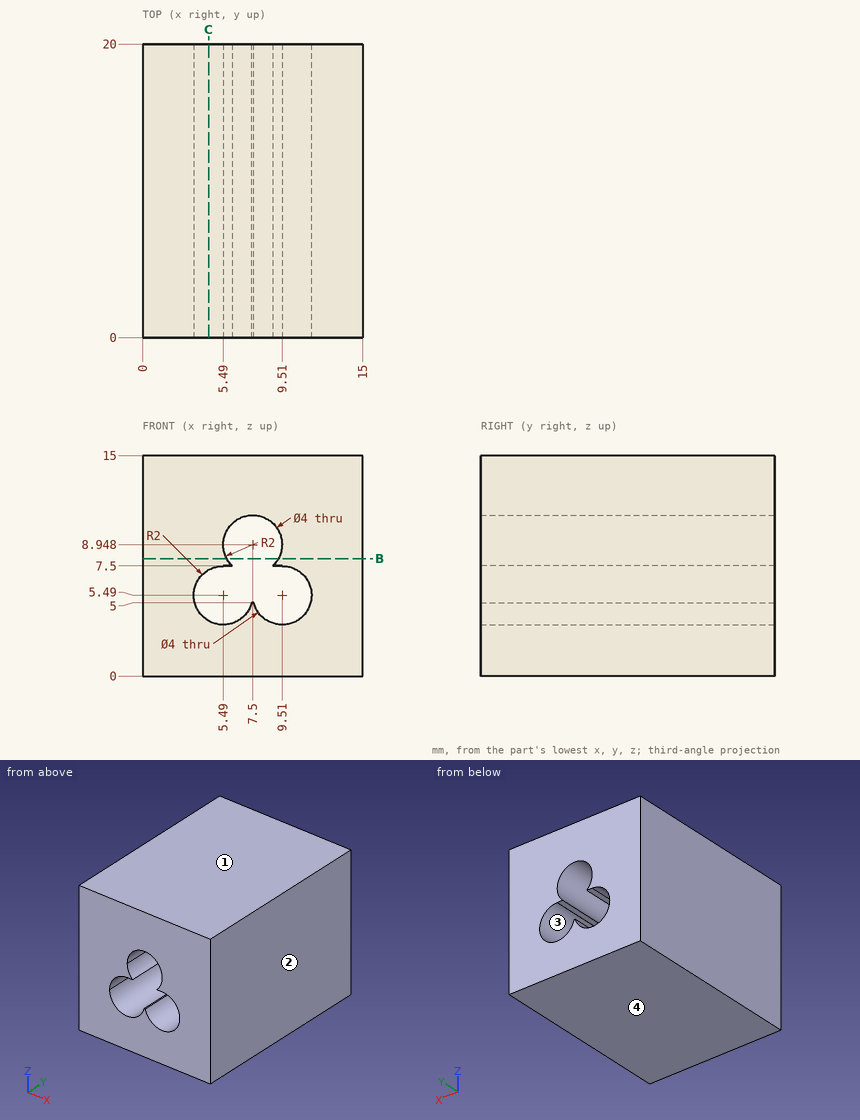
Print and shaded views of the part. All mm, measured from the part's lowest x, y and z. Round coordinates to 2 decimals unless told otherwise and drop trailing zeros. Write each loop counter-clockwise with the first axis right and the second up, starting at its lowest first coordinate (ties: lowest second). Pieces come first, ordered by that corner, then holes. Notation, with made-up numbers: (-34.75, 48) - (20.25, 48) arc R23 ccw to (20.25, 72) - close; hole circle Ø11 at (-30, -6). An arc over 180 degrees is marked (long way). Write each question's results on one line, items separated by ' | '. Start each with the question number.
Item 1: Mould opens along Z. For the marked faces 1, 2, 3 and 4 say: pulls with the +Z half, pulls with the -Z half, needs draft (parallel to the pull), parting line crosses it, or undercut.
Item 2: Wall check: L1, parallel to Z at x = 7.5, y = 17; L2, parallel to Z at x = 9.25, y = 5.25 (1 decimal); L3, parallel to X at y = 4.25, z = 4.75. Give the ranges that are in metal, low to high. Write a range as [from, to].
Item 3: Saw through at C-C (x = 4.5). Write the cut outline in (y, z).
Item 4: Saw through at B-B (z = 8). Write the cut outline in (x, y), and give its area (3 significant figures).
Results are:
1) face 1: pulls with the +Z half | face 2: needs draft | face 3: undercut | face 4: pulls with the -Z half
2) L1: z = [0, 5], [10.95, 15] | L2: z = [0, 3.5], [7.5, 8], [9.9, 15] | L3: x = [0, 3.63], [7.35, 7.65], [11.37, 15]
3) outline: (0, 0) - (20, 0) - (20, 3.75) - (0, 3.75) - close; (0, 7.23) - (20, 7.23) - (20, 15) - (0, 15) - close
4) outline: (0, 0) - (5.74, 0) - (5.74, 20) - (0, 20) - close; (9.26, 0) - (15, 0) - (15, 20) - (9.26, 20) - close | area: 230 mm²
